Geometry: see drawing. Coordinates: mm, zero at the bounding-box minimum. Give positions to 0.01 mm unless a question says otherwise; leave off trailing zeros. Write each loop counter-clockwise with the first axis right and the second up, starting at its lowest first coordinate (ties: lowest second). Pieces come first, ordered by that corner, then holes. Notation, with made-up numbers: (4.25, 6) -> (21.25, 6) arc R15 ccw to (21.25, 21) -> close; hole circle Ø3 at (-40, 8.25). An arc over 180 degrees is marked (long way). Answer as a JSON object with one key per item and string values. Group by question number.
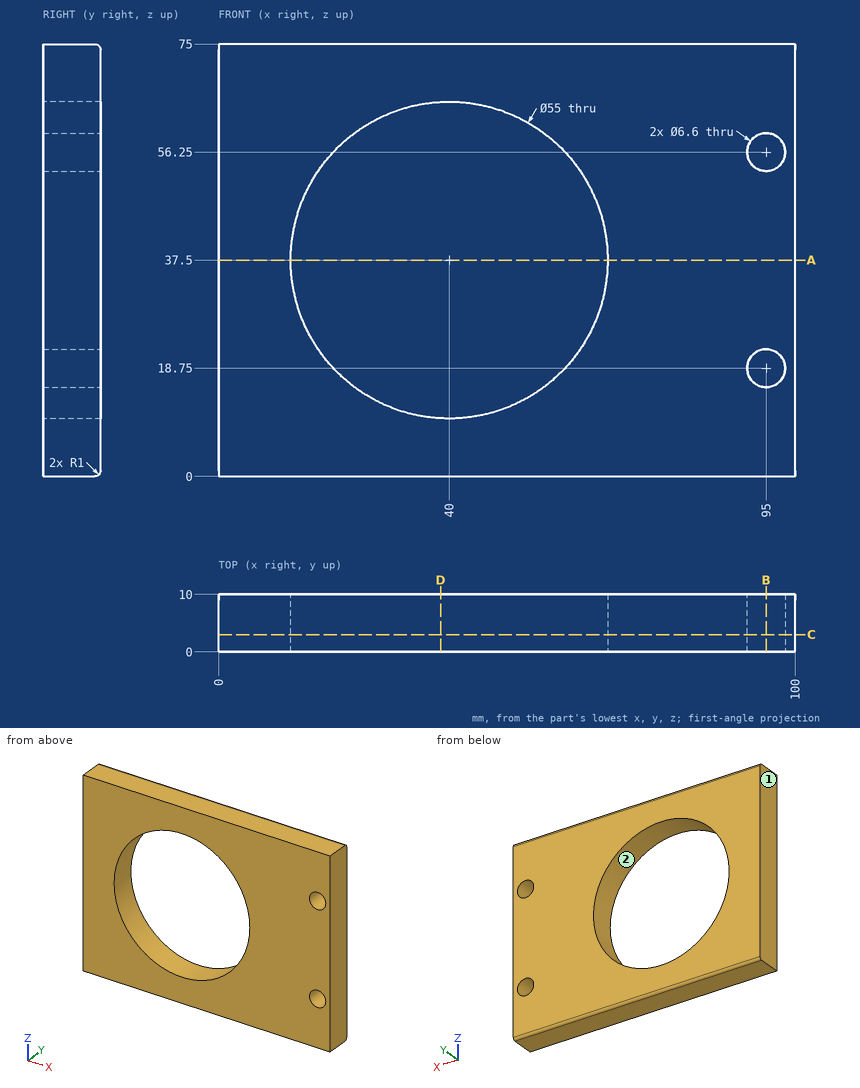
1. Section C-C (y = 3). Return the cut outline in (x, z).
2. Section B-B (x = 95). Return the cut outline in (y, z).
3. Section D-D (x = 38.5). Return the cut outline in (y, z), plus the area to 3 significant figures.
4. Section A-A (z = 37.5). Return the cut outline in (x, y), plus the area to 3 significant figures.
5. Mould query, pull axis Z, two halves, no side actions, for the marked faces 1 and 2. Classes: pulls with the +Z half, pulls with the -Z half, needs draft (parallel to the pull), parting line crosses it, or undercut.
6. Line query: line 1 (Z direction, x = 95, y = 4.25); line 2 (Z direction, x = 40, y = 2.75); line 3 (X direction, y = 2.75, z = 20.5). Output: solid intervals per line, ascending.
Working result:
{
 "1": {"outline": "(0, 0) -> (100, 0) -> (100, 75) -> (0, 75) -> close; hole circle Ø55 at (40, 37.5); hole circle Ø6.6 at (95, 18.75); hole circle Ø6.6 at (95, 56.25)"},
 "2": {"outline": "(0, 0) -> (9, 0) arc R1 ccw to (10, 1) -> (10, 15.45) -> (0, 15.45) -> close; (0, 22.05) -> (10, 22.05) -> (10, 52.95) -> (0, 52.95) -> close; (0, 59.55) -> (10, 59.55) -> (10, 74) arc R1 ccw to (9, 75) -> (0, 75) -> close"},
 "3": {"outline": "(0, 0) -> (9, 0) arc R1 ccw to (10, 1) -> (10, 10.04) -> (0, 10.04) -> close; (0, 64.96) -> (10, 64.96) -> (10, 74) arc R1 ccw to (9, 75) -> (0, 75) -> close", "area": "200 mm^2"},
 "4": {"outline": "(0, 0) -> (12.5, 0) -> (12.5, 10) -> (0, 10) -> close; (67.5, 0) -> (100, 0) -> (100, 10) -> (67.5, 10) -> close", "area": "450 mm^2"},
 "5": {"face 1": "needs draft", "face 2": "undercut"},
 "6": {"line 1": "z = 0 to 15.45, 22.05 to 52.95, 59.55 to 75", "line 2": "z = 0 to 10, 65 to 75", "line 3": "x = 0 to 18.38, 61.62 to 92.2, 97.8 to 100"}
}
